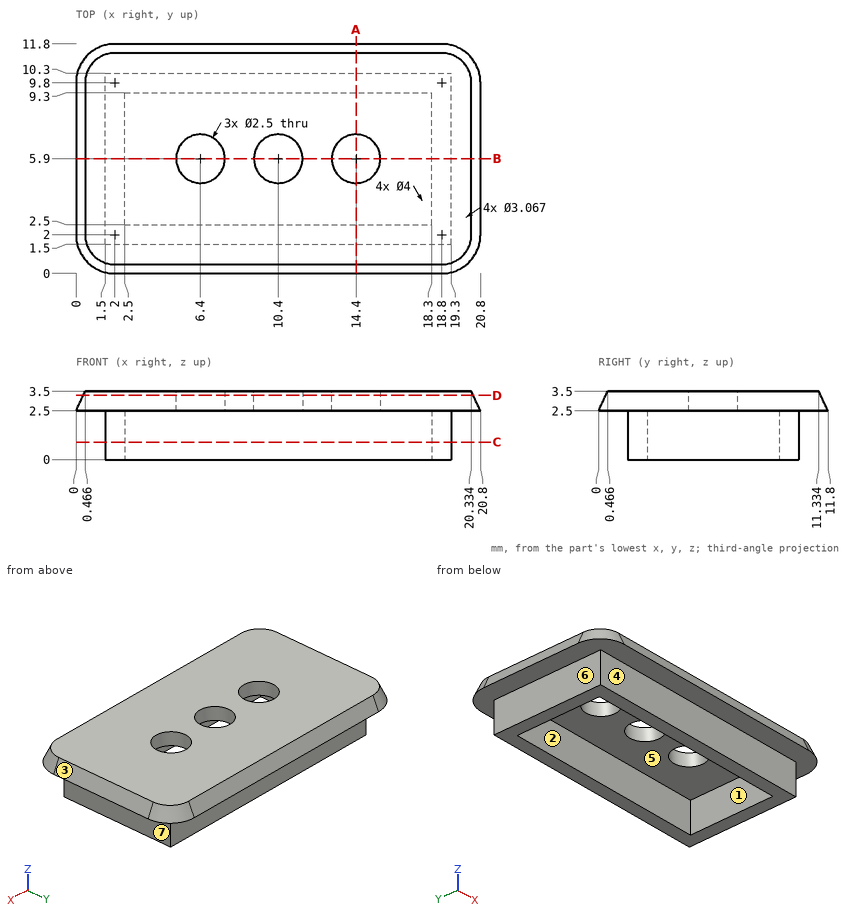
Can you work these out from the drawing? Everything is in mm from the part's minimum corner. A direction names the side the tool comes from. Coordinates: 2 decimals unless noted, no trailing zeros. Loops run counter-clockwise (first coordinate to the right, second up) from the corner with the lowest first, then second, coordinate; pieces in that order, holes last.
1) Imagine slicing it at B-B on y = 5.9. List the corners of the cut face in (x, z) for me.
2) Thinking about a two-plate mould opening in X: for the marked faces 1, 2, 3 and 4, which applies, pulls with the +X half, pulls with the -X half, needs draft (parallel to the pull), parting line crosses it, or undercut?
3) Imagine slicing it at D-D on z = 3.3. List the corners of the cut face in (x, y) for me.
4) Which directions (+Z, -Z, +X, -X, +Y, -Y) give clear straight access to the entire face, cutting with the end or side of a thin tool? Please do the marked faces 5, 6 and 7.
5) Imagine slicing it at C-C on z = 0.9. List the corners of the cut face in (x, y) for me.
6) For pin 1 (3 mm diameter, centred on x = 5, y = 5, fed in from -Z); pin 2 (2 mm diameter, centred on x = 8, z = 1, fed in from +Y); pin 3 (0.8 mm diameter, centred on x = 9, z = 2, fed in from -Y); pin 4 (4 mm diameter, centred on x = 14.4, y = 5.9, fed in from +Z), each with a flat end and sliding along its axis, tell me the tip position at first contact or that it passes through.
7) I need wall thicknesses on probe 1 along Y at (x, z) = (4.75, 2.25); probe 2 along X at (y, z) = (3.75, 1.45); probe 3 along Z at (x, y) = (18, 7). Which ranges of each line are inside material? Lowest first, please.
8) Imagine slicing it at A-A on x = 14.4. List the corners of the cut face in (y, z) for me.
Completed:
1. outline: (0, 2.5) - (1.5, 2.5) - (1.5, 0) - (2.5, 0) - (2.5, 2.5) - (5.15, 2.5) - (5.15, 3.5) - (0.47, 3.5) - close; (7.65, 2.5) - (9.15, 2.5) - (9.15, 3.5) - (7.65, 3.5) - close; (11.65, 2.5) - (13.15, 2.5) - (13.15, 3.5) - (11.65, 3.5) - close; (15.65, 2.5) - (18.3, 2.5) - (18.3, 0) - (19.3, 0) - (19.3, 2.5) - (20.8, 2.5) - (20.33, 3.5) - (15.65, 3.5) - close
2. face 1: undercut
2. face 2: undercut
2. face 3: pulls with the +X half
2. face 4: needs draft
3. outline: (0.37, 2) arc R1.63 ccw to (2, 0.37) - (18.8, 0.37) arc R1.63 ccw to (20.43, 2) - (20.43, 9.8) arc R1.63 ccw to (18.8, 11.43) - (2, 11.43) arc R1.63 ccw to (0.37, 9.8) - close; hole circle Ø2.5 at (6.4, 5.9); hole circle Ø2.5 at (10.4, 5.9); hole circle Ø2.5 at (14.4, 5.9)
4. face 5: -Z
4. face 6: -Z, -X, +Y, -Y
4. face 7: -Z, +X, +Y, -Y
5. outline: (1.5, 1.5) - (19.3, 1.5) - (19.3, 10.3) - (1.5, 10.3) - close; hole (2.5, 2.5) - (18.3, 2.5) - (18.3, 9.3) - (2.5, 9.3) - close
6. pin 1: stops at z = 2.5
6. pin 2: stops at y = 10.3
6. pin 3: stops at y = 1.5
6. pin 4: stops at z = 3.5
7. probe 1: y = 1.5 to 2.5, 9.3 to 10.3
7. probe 2: x = 1.5 to 2.5, 18.3 to 19.3
7. probe 3: z = 2.5 to 3.5
8. outline: (0, 2.5) - (1.5, 2.5) - (1.5, 0) - (2.5, 0) - (2.5, 2.5) - (4.65, 2.5) - (4.65, 3.5) - (0.47, 3.5) - close; (7.15, 2.5) - (9.3, 2.5) - (9.3, 0) - (10.3, 0) - (10.3, 2.5) - (11.8, 2.5) - (11.33, 3.5) - (7.15, 3.5) - close
